from build123d import *

# Parameters (mm, degrees)
EXTRUDE_1_DEPTH          = 10
SKETCH_2_R               = 14
SKETCH_2_R_2             = 1.45
CUT_EXTRUDE_1_DEPTH      = 10
CUT_EXTRUDE_START        = -7
SKETCH_4_R               = 3.2
SKETCH_4_R_2             = 1.45
CUT_EXTRUDE_2_DEPTH      = 7
SKETCH_4_3_W             = 43.30127019
SKETCH_4_3_H             = 7
CUT_EXTRUDE_3_DEPTH      = 4
SKETCH_4_4_R             = 1.7
CUT_EXTRUDE_4_DEPTH      = 41
EXTRUDE_START            = 3
SKETCH_5_R               = 28
SKETCH_5_R_2             = 14
SKETCH_5_R_3             = 1.426889677
SKETCH_5_R_4             = 1.45
EXTRUDE_2_DEPTH          = 3
PATTERN_CIRCULAR_1_COUNT = 3


with BuildPart() as part:
    # Sketch 1 → Extrude 1 (new body)
    with BuildSketch(Plane(origin=(0, 0, 0), x_dir=(1, 0, 0), z_dir=(0, 1, 0))):
        Polygon((43.301270189, 0), (21.650635095, 37.5), (-21.650635095, 37.5), (-43.301270189, 0), (-21.650635095, -37.5), (21.650635095, -37.5), align=None)
    extrude(amount=EXTRUDE_1_DEPTH)

    # Sketch 2 → Cut-Extrude 1 (cut)
    with BuildSketch(Plane(origin=(0, 10, 0), x_dir=(1, 0, 0), z_dir=(0, 1, 0))):
        with Locations(Location((0, 0, 0), (0, 0, 270))):
            Circle(SKETCH_2_R)
        with Locations(Location((-19, 0, 0), (0, 0, 270))):
            Circle(SKETCH_2_R_2)
        with Locations(Location((0, 19, 0), (0, 0, 270))):
            Circle(SKETCH_2_R_2)
        with Locations(Location((19, 0, 0), (0, 0, 270))):
            Circle(SKETCH_2_R_2)
        with Locations(Location((0, -19, 0), (0, 0, 270))):
            Circle(SKETCH_2_R_2)
    extrude(amount=-CUT_EXTRUDE_1_DEPTH, mode=Mode.SUBTRACT)

    # Sketch 4 → Cut-Extrude 2 (cut)
    # profile 1 of 4: a face of its own
    with BuildSketch(Plane.XZ.offset(CUT_EXTRUDE_START)):
        with Locations(Location((-19, 0, 0), (0, 0, 270))):
            Circle(SKETCH_4_R)
        with Locations(Location((-19, 0, 0), (0, 0, 90))):
            Circle(SKETCH_4_R_2, mode=Mode.SUBTRACT)
    # profile 2 of 4: a face of its own
    with BuildSketch(Plane.XZ.offset(CUT_EXTRUDE_START)):
        with Locations(Location((19, 0, 0), (0, 0, 270))):
            Circle(SKETCH_4_R)
        with Locations(Location((19, 0, 0), (0, 0, 90))):
            Circle(SKETCH_4_R_2, mode=Mode.SUBTRACT)
    # profile 3 of 4: a face of its own
    with BuildSketch(Plane.XZ.offset(CUT_EXTRUDE_START)):
        with Locations(Location((0, 19, 0), (0, 0, 270))):
            Circle(SKETCH_4_R)
        with Locations(Location((0, 19, 0), (0, 0, 90))):
            Circle(SKETCH_4_R_2, mode=Mode.SUBTRACT)
    # profile 4 of 4: a face of its own
    with BuildSketch(Plane.XZ.offset(CUT_EXTRUDE_START)):
        with Locations(Location((0, -19, 0), (0, 0, 270))):
            Circle(SKETCH_4_R)
    extrude(amount=CUT_EXTRUDE_2_DEPTH, mode=Mode.SUBTRACT)

    # Sketch 4_3 → Cut-Extrude 3 (cut)
    with BuildSketch(Plane.XZ):
        with Locations((0, -34)):
            Rectangle(SKETCH_4_3_W, SKETCH_4_3_H)
    cut_extrude_3 = extrude(amount=-CUT_EXTRUDE_3_DEPTH, mode=Mode.SUBTRACT)

    # Sketch 4_4 → Cut-Extrude 4 (cut)
    with BuildSketch(Plane.XZ):
        with Locations(Location((8, -33.5, 0), (0, 0, 90))):
            Circle(SKETCH_4_4_R)
        with Locations(Location((-8, -33.5, 0), (0, 0, 90))):
            Circle(SKETCH_4_4_R)
    cut_extrude_4 = extrude(amount=-CUT_EXTRUDE_4_DEPTH, mode=Mode.SUBTRACT)

    # Sketch 5 → Extrude 2 (add)
    with BuildSketch(Plane(origin=(0, 10, 0), x_dir=(1, 0, 0), z_dir=(0, 1, 0)).offset(EXTRUDE_START)):
        with Locations(Location((0, 0, 0), (0, 0, 270))):
            Circle(SKETCH_5_R)
        with Locations(Location((0, 0, 0), (0, 0, 270))):
            Circle(SKETCH_5_R_2, mode=Mode.SUBTRACT)
        with Locations(Location((19, 0, 0), (0, 0, 270))):
            Circle(SKETCH_5_R_3, mode=Mode.SUBTRACT)
        with Locations(Location((0, 19, 0), (0, 0, 270))):
            Circle(SKETCH_5_R_4, mode=Mode.SUBTRACT)
        with Locations(Location((-19, 0, 0), (0, 0, 270))):
            Circle(SKETCH_5_R_4, mode=Mode.SUBTRACT)
        with Locations(Location((0, -19, 0), (0, 0, 270))):
            Circle(SKETCH_5_R_4, mode=Mode.SUBTRACT)
    extrude(amount=-EXTRUDE_2_DEPTH)

    # Pattern Circular 1: Cut-Extrude 3, Cut-Extrude 4 ×3 about axis
    pattern_circular_1_axis = Axis((0, 0, 0), (0, 1, 0))
    add([cut_extrude_3.rotate(pattern_circular_1_axis, i * 360 / PATTERN_CIRCULAR_1_COUNT) for i in range(1, PATTERN_CIRCULAR_1_COUNT)], mode=Mode.SUBTRACT)
    add([cut_extrude_4.rotate(pattern_circular_1_axis, i * 360 / PATTERN_CIRCULAR_1_COUNT) for i in range(1, PATTERN_CIRCULAR_1_COUNT)], mode=Mode.SUBTRACT)


solid = part.part
The model under review builds one solid part; all positions refer to its coordinate system, in mm. A direction names the side the tool comes from. Coordinates: 2 decimals unless noted, no trailing zeros. Write each loop counter-clockwise with the first axis right and the second up, starting at its lowest first coordinate (ties: lowest second). Pieces come first, ordered by that corner, then holes. Notation, with made-up numbers: (7, 89.5) - (65, 89.5) arc R9 ccw to (65, 100.5) - close; hole circle Ø2 at (6, 82.5). An arc over 180 degrees is marked (long way). Answer as a JSON object with one key per item and string values. Group by question number.
1. Machinability: for faces 1 (the face through (-40.313, 1.972, -1.726)), 2 (the face through (19.8, 7, -1.4)), which of the approach directions +Z, -Z, +X, -X, +Y, -Y give a long, thin tool a straight path to every point of the face, cutting with its end or side? Answer none if there is none.
2. Add section D-D (x = -33). Give the boundary of the cut face in (y, z).
3. Add section A-A (x = 0). Give the number of separate pieces and of enclosed holes in the cut face, plus the area to 3 significant figures.
4. Mouldability with a two-part tool opening along X and no side actions: class faces 3 (the face through (21.651, 2, -34)), 4 (the face through (0, 5, 37.5)), 5 (the face through (32.628, 4.93, -18.488)) as pulls with the +X half, pulls with the -X half, needs draft (parallel to the pull), parting line crosses it, or undercut.
5. To check wall thickness, follow probe 1 along Z at (x, y) = (12.5, 6.5); probe 2 along Z at (x, y) = (19, 8.6); probe 3 along X at (y, z) = (8.4, -33.5). State the ranges of each line that lie inside material, in increasing order.
6. Add section B-B (y = 2.75). Give the boundary of the cut face in (x, z), plus the area to 3 significant figures.
7. Add section C-C (z = 6.5). Give the boundary of the cut face in (x, y), plus the area to 3 significant figures.
8. Clearance check with flat-ended pins moving along their axes: pin 1 Ø5 at (x, z) = (0, 19) entering from -Y; pin 2 Ø2.5 at (x, z) = (-19, 0) entering from -Y; pin 3 Ø2 at (y, z) = (9.5, 26.5) entering from -X; pin 4 Ø1 at (y, z) = (1.5, -7.5) entering from +X. State where each tip first meets the part, or that it passes through.
Findings:
{
 "1": {"face 1": "+Z, -Y", "face 2": "-Y"},
 "2": {"outline": "(0, -17.84) - (10, -17.84) - (10, 8.12) - (4, 8.12) - (4, 3.84) - (0, 3.84) - close; (4, 11.52) - (10, 11.52) - (10, 17.84) - (4, 17.84) - close"},
 "3": {"separate pieces": "4", "enclosed holes": "0", "area": "402 mm²"},
 "4": {"face 3": "undercut", "face 4": "needs draft", "face 5": "pulls with the +X half"},
 "5": {"probe 1": "-37.5 to -6.3, 6.3 to 37.5", "probe 2": "-37.5 to -1.45, 1.45 to 37.5", "probe 3": "-23.96 to -9.7, -6.3 to 6.3, 9.7 to 23.96"},
 "6": {"outline": "(-43.3, 0) - (-21.65, -37.5) - (-21.65, -30.5) - (21.65, -30.5) - (21.65, -37.5) - (43.3, 0) - (37.24, -3.5) - (15.59, 34) - (21.65, 37.5) - (-21.65, 37.5) - (-15.59, 34) - (-37.24, -3.5) - close; hole circle Ø6.4 at (-19, 0); hole circle Ø28 at (0, 0); hole circle Ø6.4 at (0, -19); hole circle Ø6.4 at (0, 19); hole circle Ø6.4 at (19, 0)", "area": "3,220 mm²"},
 "7": {"outline": "(-39.55, 4) - (-31.47, 4) - (-31.47, 0) - (-12.4, 0) - (-12.4, 13) - (-27.24, 13) - (-27.24, 10) - (-39.55, 10) - close; (12.4, 0) - (31.47, 0) - (31.47, 4) - (39.55, 4) - (39.55, 10) - (27.24, 10) - (27.24, 13) - (12.4, 13) - close", "area": "567 mm²"},
 "8": {"pin 1": "y = 7", "pin 2": "through", "pin 3": "x = -28.58", "pin 4": "x = 39.26"}
}
